Source: three-view drawing plus pictorial views. Frame: mm from the lowest corner of the part. Give positions to 0.01 mm unless a question says otherwise; leave off trailing zeros. Loops run counter-clockwise (first coordinate to the right, second up) from the corner with the lowest first, then second, coordinate; pieces in that order, holes last. Notation, with made-up numbers: M 43.5,-12 L 96.5,-12 A16 ccw 96.5,6 Z; hole C -1,14.25 d1. An arc over 180 degrees is marked long. Write item = value, one per line.
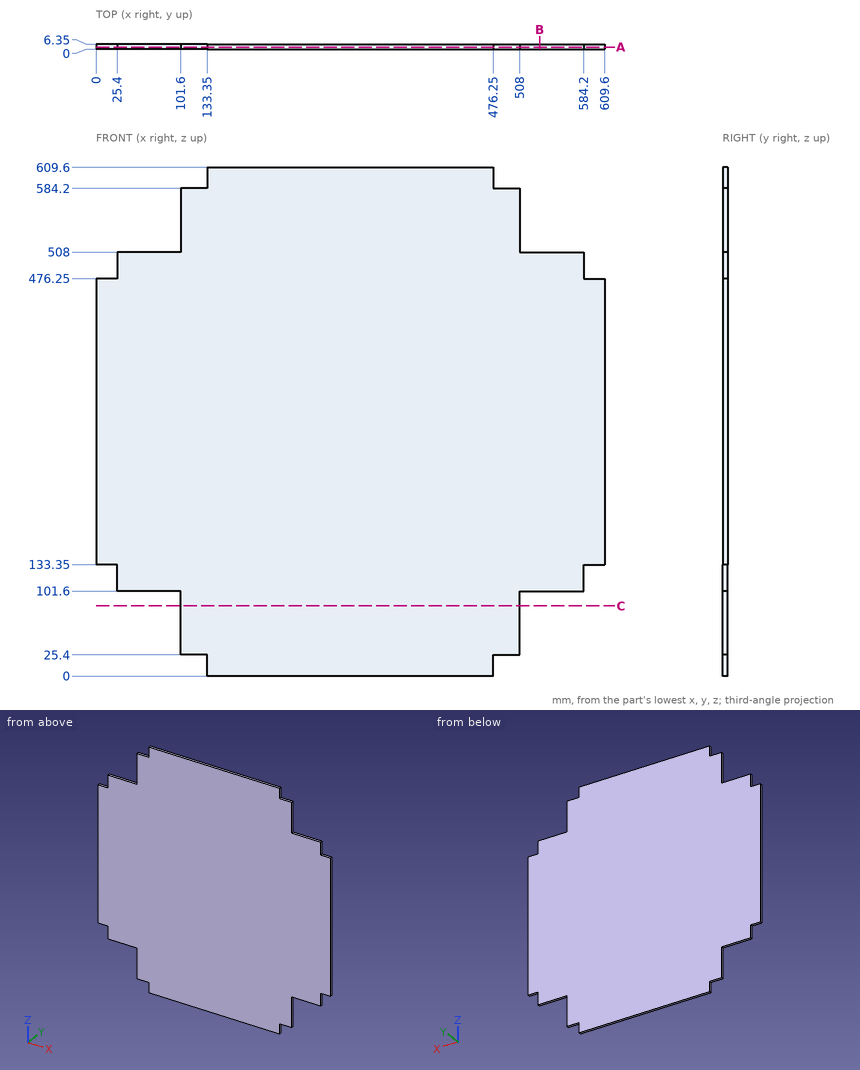
1. Material intervals for probe 1 along Z at (x, y) = (525.5, 4); probe 2 along X at (y, z) = (5.5, 503), sorted ascending. Write a range as from..to.
Derived:
probe_1 = 101.6..508
probe_2 = 25.4..584.2
2. Cut plane C-C, the plane z = 84. Return the cut outline in (x, y).
Derived:
outline = M 101.6,0 L 508,0 L 508,6.35 L 101.6,6.35 Z
3. Cut plane A-A, the plane y = 2.75. Return the cut outline in (x, z), then the cut area to 3 significant figures.
Derived:
outline = M 0,133.35 L 25.4,133.35 L 25.4,101.6 L 101.6,101.6 L 101.6,25.4 L 133.35,25.4 L 133.35,0 L 476.25,0 L 476.25,25.4 L 508,25.4 L 508,101.6 L 584.2,101.6 L 584.2,133.35 L 609.6,133.35 L 609.6,476.25 L 584.2,476.25 L 584.2,508 L 508,508 L 508,584.2 L 476.25,584.2 L 476.25,609.6 L 133.35,609.6 L 133.35,584.2 L 101.6,584.2 L 101.6,508 L 25.4,508 L 25.4,476.25 L 0,476.25 Z
area = 324,000 mm²
4. Cut plane B-B, the plane x = 531.5. Return the cut outline in (y, z), then the cut area to 3 significant figures.
Derived:
outline = M 0,101.6 L 6.35,101.6 L 6.35,508 L 0,508 Z
area = 2,580 mm²
5. First-contact query: pin 1 Ø3 at (x, y) = (596.5, 3) entering from -Z; pin 2 Ø3 at (y, z) = (2, 543.5) entering from +X; pin 3 Ø3 at (y, z) = (3, 494.5) entering from -X. Flat tips, straight axial feed; report the tip coordinate or a pass-through.
Derived:
pin_1 = 133.35
pin_2 = 508
pin_3 = 25.4
